```python
from build123d import *

# Parameters (mm, degrees)
F1_DEPTH = 1.5
F2_W     = 42
F2_H     = 25
F3_DEPTH = 60
F5_W     = 42
F5_H     = 25
F6_DEPTH = 60
F7_W     = 125
F7_H     = 15
F8_DEPTH = 25


# Not quite as in the source:
# - a pattern or mirror of a feature is missing from the dataset's text; its kind, count and spacing are read off the source's solid


with BuildPart() as f1:
    # F0 (on Top) → F1 (new body, symmetric)
    with BuildSketch(Plane.XY):
        Polygon((-77.7, -96), (0, -96), (0, 0), (324.3, 0), (324.3, 54), (-77.7, 54), align=None)
    extrude(amount=F1_DEPTH, both=True)

    # F2 (on face) → F3 (join)
    with BuildSketch(Plane.XZ.offset(96)):
        with Locations((-56.7, -14)):
            Rectangle(F2_W, F2_H)
    f3 = extrude(amount=-F3_DEPTH)

    # F3_copies: F3 across plane
    add(f3.mirror(Plane.XY))

    # F5 (on offset) → F6 (join)
    with BuildSketch(Plane.YZ.offset(274.3)):
        with Locations((33, -14)):
            Rectangle(F5_W, F5_H)
    f6 = extrude(amount=-F6_DEPTH)

    # F6_copies: F6 across plane
    add(f6.mirror(Plane.XY))

    # F7 (on face) → F8 (cut)
    with BuildSketch(Plane.XY.offset(1.5)):
        with Locations((119.8, 7.5)):
            Rectangle(F7_W, F7_H)
    extrude(amount=-F8_DEPTH, mode=Mode.SUBTRACT)


solid = f1.part
```
Geometry check sheet. Reference: the model listing, model coordinates, mm. A direction names the side the tool comes from. Coordinates: 2 decimals unless noted, no trailing zeros. Write each loop counter-clockwise with the first axis right and the second up, starting at its lowest first coordinate (ties: lowest second). Pieces come first, ordered by that corner, then holes. Notation, with made-up numbers: M 20.25,33 L 52.25,33 A30 cw 52.25,69 Z; hole C -38,-14.75 d7. An arc over 180 degrees is marked long. One line per item, written item: value. Start each with the question number.
(1) Sectioned sample at B-B, the plane x = 218. Enter the section's corners in (y, z), and give its area (3 significant figures).
(2) Sectioned sample at C-C, the plane y = -85.5. Enter the section's corners in (x, z).
(3) Sectioned sample at A-A, the plane z = 22.5. Enter the section's corners in (x, y).
(4) Scan lines: line 1 along X through (y, z) = (18.5, 17); line 2 along Z through (x, y) = (-52.5, -24); line 3 along Y through (x, z) = (252, 2). Record each from-to range of solid material in increasing order. Write a range as [from, to].
(5) Depth check by flat-ended pin: pin 1 (7.5 mm diameter, centred on y = -77, z = 17, fed in from +X); pin 2 (12.5 mm diameter, centred on y = 35.5, z = 8.5, fed in from +X); pin 3 (1.5 mm diameter, centred on x = 102.5, z = 0, fed in from -Y); pin 4 (10 mm diameter, centred on x = 36.5, y = -9.5, fed in from -Z). Enter the tip coordinate at first touch or a pass-through.
(6) Sectioned sample at D-D, the plane y = -23.5. Enter the section's corners in (x, z).
(7) Tool access check on faces 1 (the face through (-35.7, -66, -14)), 2 (the face through (214.3, 33, -14)), 3 (the face through (245, 12, 14)). Record the directions out of +Z, -Z, +X, -X, +Y, -Y that give a thin tool (end or side, any length) a straight path to the whole face; none if there is none.
Filled sheet:
1. outline: M 0,-1.5 L 12,-1.5 L 12,-26.5 L 54,-26.5 L 54,26.5 L 12,26.5 L 12,1.5 L 0,1.5 Z
1. area: 2,260 mm²
2. outline: M -77.7,-26.5 L -35.7,-26.5 L -35.7,-1.5 L 0,-1.5 L 0,1.5 L -35.7,1.5 L -35.7,26.5 L -77.7,26.5 Z
3. outline: M -77.7,-96 L -35.7,-96 L -35.7,-36 L -77.7,-36 Z; M 214.3,12 L 274.3,12 L 274.3,54 L 214.3,54 Z
4. line 1: [214.3, 274.3]
4. line 2: [-1.5, 1.5]
4. line 3: [12, 54]
5. pin 1: x = -35.7
5. pin 2: x = 274.3
5. pin 3: y = 15
5. pin 4: through
6. outline: M -77.7,-1.5 L 0,-1.5 L 0,1.5 L -77.7,1.5 Z
7. face 1: -Z, +X, +Y, -Y
7. face 2: -Z, -X, +Y, -Y
7. face 3: +Z, +X, -X, -Y
